from build123d import *

# Parameters (mm, degrees)
F0_W     = 40
F0_H     = 28
F1_DEPTH = 6
F2_R     = 1.3
F3_DEPTH = 10
F6_COUNT = 3
F7_R     = 6.5
F7_R_2   = 1.65
F8_DEPTH = 6.001


with BuildPart() as f1:
    # F0 (on Top) → F1 (new body)
    with BuildSketch(Plane.XY):
        with Locations((0, 14)):
            Rectangle(F0_W, F0_H)
    extrude(amount=F1_DEPTH)

    # F2 (on face) → F3 (cut)
    with BuildSketch(Plane(origin=(-20, 0, 0), x_dir=(0, -1, 0), z_dir=(-1, 0, 0))):
        with Locations((-22, 3)):
            Circle(F2_R)
    extrude(amount=-F3_DEPTH, mode=Mode.SUBTRACT)

    # F4: F1 across plane


with BuildPart() as f1_1:
    add(f1.part)
    add(f1.part.mirror(Plane.YZ), mode=Mode.INTERSECT)

    # F6: F1 ×3 about axis
    f6_axis = Axis((0, 0, 8.396655), (0, 0, 1))


with BuildPart() as f1_2:
    add(f1_1.part)
    for i in range(1, F6_COUNT):
        add(f1_1.part.rotate(f6_axis, i * 360 / F6_COUNT))

    # F7 (on face) → F8 (cut, through all)
    with BuildSketch(Plane.XY.offset(6)):
        Circle(F7_R)
        with Locations((0, 12.5)):
            Circle(F7_R_2)
        with Locations((10.825318, 6.25)):
            Circle(F7_R_2)
        with Locations((10.825318, -6.25)):
            Circle(F7_R_2)
        with Locations((0, -12.5)):
            Circle(F7_R_2)
        with Locations((-10.825318, 6.25)):
            Circle(F7_R_2)
        with Locations((-10.825318, -6.25)):
            Circle(F7_R_2)
    extrude(amount=-F8_DEPTH, mode=Mode.SUBTRACT)


solid = f1_2.part
For this review, take the finished solid that the model builds, in its own axes (mm). A direction names the side the tool comes from. Give positions to 0.01 mm unless a question says otherwise; leave off trailing zeros. Loops run counter-clockwise (first coordinate to the right, second up) from the corner with the lowest first, then second, coordinate; pieces in that order, holes last.
Item 1: Draft analysis for pull direction Z (two halves, no side actions). For faces 5 (the flat face through (7, 4, 0)), 6 (the cylindrical face through (12.35, -6.88, 3.04)), 7 (the flat face through (-24.07, -2.35, 3.02)), state which applies: +Z half, -Z half, draft (parallel to the pull), parting line (faces both ways), or undercut.
Item 2: Tool access review of faces 1 (the flat face through (20, 20, 3)), 2 (the flat face through (7.025, -27.15, 2.958)), 3 (the flat face through (-10, 22, 3)), 4 (the flat face through (-20, 20, 3)): name each direction out of +Z, -Z, +X, -X, +Y, -Y from which nothing blocks a thin tool from reaching the whole face with its end or side.
Item 3: Take a section at A-A, the plane y = 12.5. State the section outline as (x, z) points, and give its area (3 significant figures).
Item 4: Take a section at C-C, the plane x = 3. State the section outline as (y, z) points.
Item 5: Insertion check: pin 1 (12 mm diameter, centred on x = 25, y = 16.5, fed in from +Z); pin 2 (1.3 mm diameter, centred on y = 22, z = 2.5, fed in from +X); pin 3 (1.5 mm diameter, centred on y = -4, z = 2, fed in from -X); pin 4 (0.8 mm diameter, centred on y = 21.5, z = 3, fed in from -X). Each pin has a flat end and moves straight along its axis. Give the tip position at first contact, or say it passes through.
Item 6: Take a section at D-D, the plane x = 16. State the section outline as (y, z) points.
Item 7: Take a section at B-B, the plane z = 5.15. State the section outline as (x, y) points, and give its area (3 significant figures).
Item 8: For line 1 along Y through (x, z) = (0, 4.2); line 2 along Z through (x, y) = (-17, 22); line 3 along X through (y, z) = (-14, 3.55), list the stretches that pass through material, from the lowest coordinate up.
Calculated:
1. face 5: -Z half
1. face 6: draft
1. face 7: undercut
2. face 1: +Z, -Z, +X, +Y
2. face 2: +Z, -Z, -Y
2. face 3: -X
2. face 4: +Z, -Z, -X, +Y
3. outline: (-20, 0) - (-1.65, 0) - (-1.65, 6) - (-20, 6) - close; (1.65, 0) - (20, 0) - (20, 6) - (1.65, 6) - close
3. area: 220 mm2
4. outline: (-24.83, 0) - (-5.77, 0) - (-5.77, 6) - (-24.83, 6) - close; (5.77, 0) - (28, 0) - (28, 6) - (5.77, 6) - close
5. pin 1: stops at z = 6
5. pin 2: stops at x = 10
5. pin 3: stops at x = -30.46
5. pin 4: stops at x = -10
6. outline: (-28.29, 0) - (28, 0) - (28, 6) - (-28.29, 6) - close; hole circle Ø2.6 at (22, 3)
7. outline: (-34.25, 3.32) - (-14.25, -31.32) - (0, -23.09) - (14.25, -31.32) - (34.25, 3.32) - (20, 11.55) - (20, 28) - (-20, 28) - (-20, 11.55) - close; hole circle Ø3.3 at (-10.83, -6.25); hole circle Ø3.3 at (-10.83, 6.25); hole circle Ø13 at (0, 0); hole circle Ø3.3 at (0, -12.5); hole circle Ø3.3 at (0, 12.5); hole circle Ø3.3 at (10.83, -6.25); hole circle Ø3.3 at (10.83, 6.25)
7. area: 2,480 mm2
8. line 1: y = -23.09 to -14.15, -10.85 to -6.5, 6.5 to 10.85, 14.15 to 28
8. line 2: z = 0 to 1.7, 4.3 to 6
8. line 3: x = -24.25 to -0.69, 0.69 to 24.25
